Read the model definition and answer for the solid it produces. Units are mm, in the model's axes. Give positions to 0.01 mm unless a question says otherwise; leave off trailing zeros. Order: outer loops, then holes, each group sorted by start corner. A loop starts at its lowest first (then second) coordinate and runs counter-clockwise, first axis right, second up. Notation, with made-up numbers: (-34.75, -29) - (2.25, -29) arc R11 ccw to (2.25, -8) - close; hole circle Ø4 at (29, 80.5). An arc over 180 degrees is marked (long way). One line per item, written item: value. Start each with the question number.
```python
from build123d import *

# Parameters (mm, degrees)
EXTRUDE_1_DEPTH     = 645
SKETCH_2_R          = 1.5
CUT_EXTRUDE_2_DEPTH = 646.305354077
SKETCH_3_W          = 2
SKETCH_3_H          = 2
EXTRUDE_2_DEPTH     = 645


with BuildPart() as part:
    # Эскиз1 → Бобышка-Вытянуть1 (new body)
    with BuildSketch(Plane.XY):
        Polygon((0, 0), (0, 13), (-2, 13), (-2, -2), (13, -2), (13, 0), align=None)
    extrude(amount=-EXTRUDE_1_DEPTH)

    # Эскиз2 → Вырез-Вытянуть2 (cut, through all)
    with BuildSketch(Plane.ZY.offset(2)):
        with Locations(Location((-23.79, 4, 0), (0, 0, 270))):
            Circle(SKETCH_2_R)
        with Locations(Location((-16.29, 9, 0), (0, 0, 270))):
            Circle(SKETCH_2_R)
        with Locations(Location((-628.71, 9, 0), (0, 0, 270))):
            Circle(SKETCH_2_R)
        with Locations(Location((-621.21, 4, 0), (0, 0, 270))):
            Circle(SKETCH_2_R)
    extrude(amount=-CUT_EXTRUDE_2_DEPTH, mode=Mode.SUBTRACT)

    # Эскиз3 → Бобышка-Вытянуть2 (add)
    with BuildSketch(Plane(origin=(0, 0, -645), x_dir=(-1, 0, 0), z_dir=(0, 0, -1))):
        with Locations((-14, -1)):
            Rectangle(SKETCH_3_W, SKETCH_3_H)
        with Locations((1, 14)):
            Rectangle(SKETCH_3_W, SKETCH_3_H)
    extrude(amount=-EXTRUDE_2_DEPTH)


solid = part.part
```
1) Section A-A on x = 4.75 is taken. Write down the section's boundary in (y, z).
2) Find the intervals of material crossed by probe 1 along Z at (x, y) = (-0.5, 9); probe 2 along Z at (x, y) = (-0.7, 4); probe 3 along Y at (x, z) = (1.75, -232), in increasing order. Write a range as from..to.
3) The mould has two halves that part along Y. Classify faces 1 (the flat face through (7, -2, -327)), 2 (the flat face through (8, 0, -327)), 3 (the flat face through (0, 7, -318)): +Y half, -Y half, draft (parallel to the pull), parting line (faces both ways), or undercut.
4) Each of these flat-tipped pins is pushed along its axis until it touches: pin 1 (2.5 mm diameter, centred on y = 9, z = -16.29, fed in from -X); pin 2 (3 mm diameter, centred on x = 2.5, z = -371, fed in from +Y); pin 3 (4 mm diameter, centred on y = 4, z = -23.79, fed in from -X); pin 4 (1.5 mm diameter, centred on y = 11.5, z = -357.5, fed in from +X). Where does it stop, or does it pass through?
5) Section B-B on z = -488 is taken. Write down the section's boundary in (x, y), plus the area to 3 significant figures.
Solved:
1. outline: (-2, -645) - (0, -645) - (0, 0) - (-2, 0) - close
2. probe 1: z = -645..-630.21, -627.21..-17.79, -14.79..0
2. probe 2: z = -645..-622.71, -619.71..-25.29, -22.29..0
2. probe 3: y = -2..0
3. face 1: -Y half
3. face 2: +Y half
3. face 3: draft
4. pin 1: passes through
4. pin 2: stops at y = 0
4. pin 3: stops at x = -2
4. pin 4: stops at x = 0
5. outline: (-2, -2) - (15, -2) - (15, 0) - (0, 0) - (0, 15) - (-2, 15) - close
5. area: 64.0 mm2
